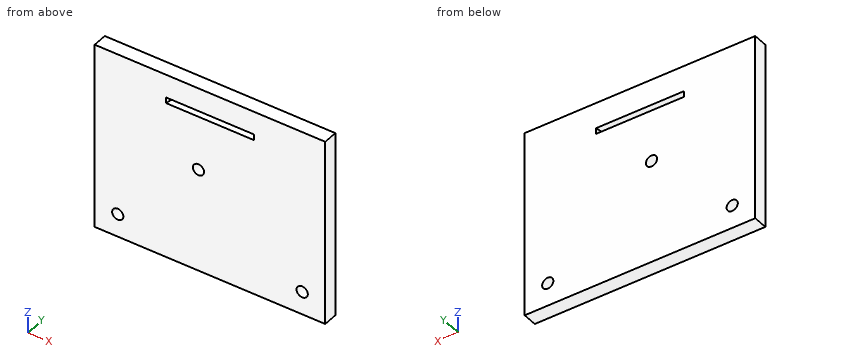
from build123d import *

# Parameters (mm, degrees)
ESQUISSE1_W                  = 80
ESQUISSE1_H                  = 65
BOSS_EXTRU_1_DEPTH           = 5
D_GAGEMENT_M3_51_D           = 3.9
ESQUISSE7_W                  = 30.5
ESQUISSE7_H                  = 2
ENL_V_MAT_EXTRU_1_DEPTH      = 5.924038765
ENL_V_MAT_EXTRU_1_DEPTH_BACK = 12.287131548


with BuildPart() as part:
    # Esquisse1 → Boss.-Extru.1 (new body)
    with BuildSketch(Plane(origin=(0, 0, 0), x_dir=(1, 0, 0), z_dir=(0, 1, 0))):
        with Locations((40, 32.5)):
            Rectangle(ESQUISSE1_W, ESQUISSE1_H)
    extrude(amount=BOSS_EXTRU_1_DEPTH)

    # Dégagement M3.51 (through all)
    with Locations(Plane(origin=(0, 5, 0), x_dir=(1, 0, 0), z_dir=(0, 1, 0))):
        with Locations((8, 57), (36, 29), (72, 57)):
            Hole(D_GAGEMENT_M3_51_D / 2)

    # Esquisse7 → Enlèv. mat.-Extru.1 (cut, two sides)
    with BuildSketch(Plane(origin=(0, 4.849231552, -0.855050358), x_dir=(-1, 0, 0), z_dir=(0, -0.984807753, 0.173648178))) as enl_v_mat_extru_1_sk:
        with Locations((-40, 8.964644395)):
            Rectangle(ESQUISSE7_W, ESQUISSE7_H)
    extrude(amount=ENL_V_MAT_EXTRU_1_DEPTH, mode=Mode.SUBTRACT)
    extrude(enl_v_mat_extru_1_sk.sketch, amount=-ENL_V_MAT_EXTRU_1_DEPTH_BACK, mode=Mode.SUBTRACT)


solid = part.part
Input: part model. Units: mm. Frame: model coordinates. Round coordinates to 2 decimals unless told otherwise and drop trailing zeros. Loops run counter-clockwise (first coordinate to the right, second up) from the corner with the lowest first, then second, coordinate; pieces in that order, holes last. Notation, with made-up numbers: M 43,47.5 L 85,47.5 A8 cw 85,51.5 Z; hole C 26.5,-6.75 d3. An arc over 180 degrees is marked long. Answer as CSV lines item,"result". Start each with the question number.
(1) Section A-A, the plane z = -29. Output: boundary loops of the cut face in (x, y), plus the area to 4 significant figures.
(2) Line query: line 1 (X direction, y = 3.65, z = -57); line 2 (X direction, y = 1.55, z = -29); line 3 (Z direction, x = 72, y = 3.8). Output: solid intervals per line, ascending. Write a range as [from, to].
(3) Section C-C, the plane z = -57. Output: boundary loops of the cut face in (x, y).
(4) Section B-B, the plane x = 8. Output: boundary loops of the cut face in (y, z), plus the area to 4 significant figures.
(5) Section D-D, the plane x = 36. Output: boundary loops of the cut face in (y, z).
(6) First-contact query: pin 1 (2.5 mm diameter, centred on x = 8, z = -57, fed in from -Y). Flat tip, straight axial feed; report the tip coordinate or a pass-through.
Values found:
1,outline,"M 0,0 L 34.05,0 L 34.05,5 L 0,5 Z; M 37.95,0 L 80,0 L 80,5 L 37.95,5 Z"
1,area,"380.5 mm²"
2,line 1,"x = [0, 6.05], [9.95, 70.05], [73.95, 80]"
2,line 2,"x = [0, 34.05], [37.95, 80]"
2,line 3,"z = [-65, -58.95], [-55.05, 0]"
3,outline,"M 0,0 L 6.05,0 L 6.05,5 L 0,5 Z; M 9.95,0 L 70.05,0 L 70.05,5 L 9.95,5 Z; M 73.95,0 L 80,0 L 80,5 L 73.95,5 Z"
4,outline,"M 0,-65 L 5,-65 L 5,-58.95 L 0,-58.95 Z; M 0,-55.05 L 5,-55.05 L 5,0 L 0,0 Z"
4,area,"305.5 mm²"
5,outline,"M 0,-65 L 5,-65 L 5,-30.95 L 0,-30.95 Z; M 0,-27.05 L 5,-27.05 L 5,-11 L 0,-10.12 Z; M 0,-8.09 L 5,-8.97 L 5,0 L 0,0 Z"
6,pin 1,"passes through"
